```python
from build123d import *

# Parameters (mm, degrees)
SKETCH1_W               = 730
SKETCH1_H               = 150
BASE_FLANGE1_DEPTH      = 2.5
EDGE_FLANGE1_DEPTH      = 730
EDGE_FLANGE1_BEND_DEPTH = 730
SKETCH13_R              = 22.5
CUT_EXTRUDE2_DEPTH      = 10
CUT_EXTRUDE3_DEPTH      = 396.173746598
CUT_EXTRUDE3_DEPTH_BACK = 396.173746598
SKETCH14_W              = 631.337566112
SKETCH14_H              = 273.157514278
CUT_EXTRUDE4_DEPTH      = 396.173746598
CUT_EXTRUDE4_DEPTH_BACK = 396.173746598
CUT_EXTRUDE5_DEPTH      = 408.87885472


# Sheet-metal steps are written as plain solids
with BuildPart() as part:
    # Sketch1 → Base-Flange1 (new body)
    with BuildSketch(Plane(origin=(0, 0, 0), x_dir=(0, 0, -1), z_dir=(1, 0, 0))):
        Rectangle(SKETCH1_W, SKETCH1_H)
    extrude(amount=-BASE_FLANGE1_DEPTH)

    # Edge-Flange1 section (across the edge) → Edge-Flange1 (add)
    with BuildSketch(Plane(origin=(-2.5, 75.2, 365), x_dir=(0, -1, 0), z_dir=(0, 0, -1))):
        with BuildLine():
            Line((-2.5, 0.2), (-2.5, 127.5))
            Line((-2.5, 127.5), (0, 127.5))
            Line((0, 127.5), (0, 0.2))
            ThreePointArc((0, 0.2), (0.058578644, 0.058578644), (0.2, 0))
            Line((0.2, 0), (0.2, -2.5))
            ThreePointArc((0.2, -2.5), (-1.709188309, -1.709188309), (-2.5, 0.2))
        make_face()
    extrude(amount=EDGE_FLANGE1_DEPTH)

    # Edge-Flange1 section 2 (across the edge) → Edge-Flange1 bend (add)
    with BuildSketch(Plane(origin=(-2.5, -75.2, -365), x_dir=(0, 1, 0), z_dir=(0, 0, 1))):
        with BuildLine():
            Line((-2.5, 0.2), (-2.5, 127.5))
            Line((-2.5, 127.5), (0, 127.5))
            Line((0, 127.5), (0, 0.2))
            ThreePointArc((0, 0.2), (0.058578644, 0.058578644), (0.2, 0))
            Line((0.2, 0), (0.2, -2.5))
            ThreePointArc((0.2, -2.5), (-1.709188309, -1.709188309), (-2.5, 0.2))
        make_face()
    extrude(amount=EDGE_FLANGE1_BEND_DEPTH)

    # Sketch13 → Cut-Extrude2 (cut)
    with BuildSketch(Plane(origin=(0, 0, 0), x_dir=(0, 0, -1), z_dir=(1, 0, 0))):
        with Locations((265, 0)):
            Circle(SKETCH13_R)
        with Locations((-290, 0)):
            Circle(SKETCH13_R)
    extrude(amount=-CUT_EXTRUDE2_DEPTH, mode=Mode.SUBTRACT)

    # Sketch14 → Cut-Extrude3 (cut, two sides: drawn at the far end of the back side and taken through both)
    with BuildSketch(Plane(origin=(0, 0, 0), x_dir=(0, 0, -1), z_dir=(1, 0, 0)).offset(-CUT_EXTRUDE3_DEPTH_BACK)):
        with Locations((-126.629311255, -14.019673746)):
            Rectangle(SKETCH14_W, SKETCH14_H)
    extrude(amount=CUT_EXTRUDE3_DEPTH + CUT_EXTRUDE3_DEPTH_BACK, mode=Mode.SUBTRACT)

    # Sketch15 → Cut-Extrude4 (cut, two sides: drawn at the far end of the back side and taken through both)
    with BuildSketch(Plane(origin=(0, 0, 0), x_dir=(0, 0, -1), z_dir=(1, 0, 0)).offset(-CUT_EXTRUDE4_DEPTH_BACK)):
        with BuildLine():
            Line((302.266550641, 80.822052704), (310.532003477, 105.351783703))
            Line((310.532003477, 105.351783703), (400.668447303, 94.566226322))
            Line((400.668447303, 94.566226322), (380.252927975, -108.048173048))
            Line((380.252927975, -108.048173048), (291.286888445, -85.029403714))
            ThreePointArc((291.286888445, -85.029403714), (353.805609642, -5.879089735), (302.266550641, 80.822052704))
        make_face()
    extrude(amount=CUT_EXTRUDE4_DEPTH + CUT_EXTRUDE4_DEPTH_BACK, mode=Mode.SUBTRACT)

    # Sketch17 → Cut-Extrude5 (cut, through all)
    with BuildSketch(Plane(origin=(0, 77.7, 0), x_dir=(1, 0, 0), z_dir=(0, 1, 0))):
        with BuildLine():
            Line((-118.819244886, 354.751470834), (-213.837944087, 354.751470834))
            Line((-213.837944087, 354.751470834), (-213.837944087, 158.380448287))
            Line((-213.837944087, 158.380448287), (-29.613553222, 158.380448287))
            ThreePointArc((-29.613553222, 158.380448287), (-63.53464157, 261.418373894), (-118.819244886, 354.751470834))
        make_face()
    extrude(amount=-CUT_EXTRUDE5_DEPTH, mode=Mode.SUBTRACT)


solid = part.part
```
Input: part model. Units: mm. Frame: model coordinates. A direction names the side the tool comes from. Give positions to 0.01 mm unless a question says otherwise; leave off trailing zeros. Loops run counter-clockwise (first coordinate to the right, second up) from the corner with the lowest first, then second, coordinate; pieces in that order, holes last. Notation, with made-up numbers: (-20.75, 54.5) -> (27.25, 54.5) arc R15 cw to (27.25, 67.5) -> close; hole circle Ø3 at (75.5, 43). An arc over 180 degrees is marked (long way). Use a Markdown table: item, result.
Q1. Pull-direction query (Y, two-part tool) for faces 1 (the cylindrical face through (-2, 0, -354)), 2 (the cylindrical face through (-1.23, 6.76, -286.46)), 3 (the flat face through (-2, 0, -189.039)); classes: pulls with the +Y half, pulls with the -Y half, needs draft (parallel to the pull), parting line crosses it, or undercut.
Entries:
| item | result |
|---|---|
| face 1 | parting line crosses it |
| face 2 | undercut |
| face 3 | needs draft |
Q2. First-contact query: P1, Ø5, axis at y = -14, z = -277, coming from the -X side; P2, Ø8, axis at y = -34.5, z = -271, coming from the -X side. Flat tips, straight axial feed; report the tip coordinate or a pass-through.
Entries:
| item | result |
|---|---|
| P1 | passes through |
| P2 | stops at x = -2.5 |
Q3. Ray query, probe 1 along Y at (x, z) = (-14.5, -256); probe 2 along X at (y, z) = (-47, -296.5); probe 3 along Y at (x, z) = (-0.85, -265). Return the intervals inside material, ascending. Write a range as from..to.
Entries:
| item | result |
|---|---|
| probe 1 | y = -77.7..-75.2, 75.2..77.7 |
| probe 2 | x = -2.5..0 |
| probe 3 | y = -76.97..-22.5, 22.5..76.97 |
Q4. Section query D-D, the plane z = -221. Return the cut outline in (x, y), plus the area to 3 significant figures.
Entries:
| item | result |
|---|---|
| outline | (-47.25, -77.7) -> (-2.7, -77.7) arc R2.7 ccw to (0, -75) -> (0, 75) arc R2.7 ccw to (-2.7, 77.7) -> (-47.25, 77.7) -> (-47.25, 75.2) -> (-2.7, 75.2) arc R0.2 cw to (-2.5, 75) -> (-2.5, -75) arc R0.2 cw to (-2.7, -75.2) -> (-47.25, -75.2) -> close |
| area | 609 mm² |
Q5. Access query for faces 4 (the flat face through (-37, -75.2, -265)), 5 (the flat face through (-35, -77.7, -263)). Directions: +Z, -Z, +X, -X, +Y, -Y. A direction counts if a zero-diameter tool reaches every point of the face in a straight line with its end or side. Return the directions, or none.
Entries:
| item | result |
|---|---|
| face 4 | +Z, -Z, -X |
| face 5 | +Z, -Z, +X, -X, -Y |
Q6. Section query A-A, the plane y = 0. Return the cut outline in (x, z), plus the area to 3 significant figures.
Entries:
| item | result |
|---|---|
| outline | (-2.5, -354) -> (0, -354) -> (0, -287.5) -> (-2.5, -287.5) -> close; (-2.5, -242.5) -> (0, -242.5) -> (0, -189.04) -> (-2.5, -189.04) -> close |
| area | 300 mm² |
Q7. Section query C-C, the plane z = -265. Return the cut outline in (x, y).
Entries:
| item | result |
|---|---|
| outline | (-65.18, -77.7) -> (-2.7, -77.7) arc R2.7 ccw to (0, -75) -> (0, -22.5) -> (-2.5, -22.5) -> (-2.5, -75) arc R0.2 cw to (-2.7, -75.2) -> (-65.18, -75.2) -> close; (-65.18, 75.2) -> (-2.7, 75.2) arc R0.2 cw to (-2.5, 75) -> (-2.5, 22.5) -> (0, 22.5) -> (0, 75) arc R2.7 ccw to (-2.7, 77.7) -> (-65.18, 77.7) -> close |
Q8. Section query B-B, the plane x = -22.5. Return the cut outline in (y, z).
Entries:
| item | result |
|---|---|
| outline | (-77.7, -308.4) arc R89 ccw to (-75.2, -312.6) -> (-75.2, -189.04) -> (-77.7, -189.04) -> close; (75.2, -312.6) arc R89 ccw to (77.7, -308.4) -> (77.7, -189.04) -> (75.2, -189.04) -> close |
